Can you work these out from the model? Positions are in its coordinate system, mm. Face numbers are marked on the shaded views. A direction names the side the tool comes from. Round coordinates to 2 decimals unless told otherwise and drop trailing zeros. Write each loop counter-clockwise with the first axis right and the second up, starting at its lowest first coordinate (ties: lowest second). Pieces come first, ordered by that corner, then holes.
Q1. Please list where these lines run through material, in increasing order: line 1 along X through (y, z) = (1.25, 11); line 2 along Z through (x, y) = (15, 1.05); line 3 along Y through (x, z) = (-12.5, 11.5).
Q2. For the marked faces 1, 2 and 3, which set-ups out of +Z, -Z, +X, -X, +Y, -Y let a thin tool reach every point of the face, with its end or its side?
Q3. I'm going to push flat-ended pins straight in: pin 1 Ø2.5 at (x, y) = (1.5, 4.5) entering from +Z (3 decimals); pin 2 Ø4 at (y, z) = (5.5, -0.5) entering from -X (3 decimals); pin 3 Ø4 at (x, y) = (3, 4) entering from -Z (3 decimals); pin 4 Ø2.5 at (x, z) = (15, -11) entering from +Y. Where does each tip first touch, or does it pass through?
Q4. If we section it at C-C (y = 6.75): Please give me the cut outline in (x, z) (3 decimals), plus the area to 3 significant figures.
Q5. If we section it at B-B (z = -4.5): Please give me the cut outline in (x, y) (3 decimals), plus the area to 3 significant figures.
Q6. If we section it at A-A (x = -2): Please give me the cut outline in (y, z) (3 decimals).
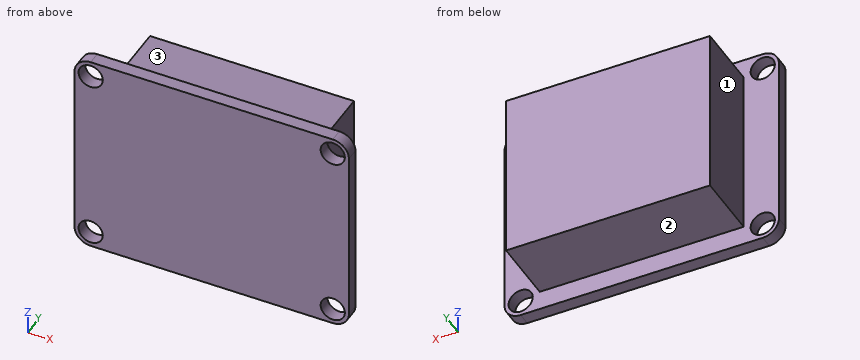
from build123d import *

# Parameters (mm, degrees)
SKETCH1_W               = 34
SKETCH1_H               = 26
BOSS_EXTRUDE1_DEPTH     = 1.6
FILLET1_R               = 2
SKETCH4_W               = 25.27
SKETCH4_H               = 21.15
BOSS_EXTRUDE3_DEPTH     = 8.19
CUT_EXTRUDE1_DEPTH      = 23.914539053
CUT_EXTRUDE1_DEPTH_BACK = 23.914539053
SKETCH5_R               = 1.5


with BuildPart() as part:
    # Sketch1 → Boss-Extrude1 (new body)
    with BuildSketch(Plane(origin=(0, 0, 0), x_dir=(1, 0, 0), z_dir=(0, 1, 0))):
        Rectangle(SKETCH1_W, SKETCH1_H)
    extrude(amount=BOSS_EXTRUDE1_DEPTH)

    # Fillet1
    fillet1_edges = [part.edges().sort_by_distance(p)[0] for p in [
        (-17, 0.8, -13),
        (17, 0.8, -13),
        (17, 0.8, 13),
        (-17, 0.8, 13),
    ]]
    fillet(fillet1_edges, radius=FILLET1_R)

    # Sketch4 → Boss-Extrude3 (add)
    with BuildSketch(Plane(origin=(0, 1.6, 0), x_dir=(1, 0, 0), z_dir=(0, 1, 0))):
        Rectangle(SKETCH4_W, SKETCH4_H)
    extrude(amount=BOSS_EXTRUDE3_DEPTH)

    # Sketch5 → Cut-Extrude1 (cut, two sides: drawn at the far end of the back side and taken through both)
    with BuildSketch(Plane(origin=(0, 1.6, 0), x_dir=(1, 0, 0), z_dir=(0, 1, 0)).offset(-CUT_EXTRUDE1_DEPTH_BACK)):
        with Locations(Location((15, 11, 0), (0, 0, 270))):
            Circle(SKETCH5_R)
        with Locations(Location((15, -11, 0), (0, 0, 270))):
            Circle(SKETCH5_R)
        with Locations(Location((-15, -11, 0), (0, 0, 270))):
            Circle(SKETCH5_R)
        with Locations(Location((-15, 11, 0), (0, 0, 270))):
            Circle(SKETCH5_R)
    extrude(amount=CUT_EXTRUDE1_DEPTH + CUT_EXTRUDE1_DEPTH_BACK, mode=Mode.SUBTRACT)


solid = part.part
A:
1. line 1: x = -17 to -16.5, -13.5 to 13.5, 16.5 to 17
1. line 2: z = -13 to -12.5, -9.5 to 9.5, 12.5 to 13
1. line 3: y = 0 to 1.6
2. face 1: +Z, -Z, -X, +Y
2. face 2: -Z, +X, -X, +Y
2. face 3: +Z, +X, -X, +Y
3. pin 1: stops at z = 10.575
3. pin 2: stops at x = -12.635
3. pin 3: stops at z = -10.575
3. pin 4: passes through
4. outline: (-12.635, -10.575) - (12.635, -10.575) - (12.635, 10.575) - (-12.635, 10.575) - close
4. area: 534 mm2
5. outline: (-17, 0) - (17, 0) - (17, 1.6) - (12.635, 1.6) - (12.635, 9.79) - (-12.635, 9.79) - (-12.635, 1.6) - (-17, 1.6) - close
5. area: 261 mm2
6. outline: (0, -13) - (1.6, -13) - (1.6, -10.575) - (9.79, -10.575) - (9.79, 10.575) - (1.6, 10.575) - (1.6, 13) - (0, 13) - close
